from build123d import *

# Parameters (mm, degrees)
F1_DEPTH  = 150
F2_R      = 13.5859557656
F3_DEPTH  = 30
F3_FACE_R = 13.5859557656
F4_DEPTH  = 15
F4_TAPER  = -45


with BuildPart() as f1:
    # F0 (on Front) → F1 (new body)
    with BuildSketch(Plane.XZ):
        Polygon((-13.63390591, 4.962335928), (-13.63390591, -4.962335928), (-7.2544498107, -12.5650756531), (2.5194439792, -14.2884768348), (11.1144619307, -9.3261409068), (14.5088996214, 0), (11.1144619307, 9.3261409068), (2.5194439792, 14.2884768348), (-7.2544498107, 12.5650756531), align=None)
    extrude(amount=F1_DEPTH)

    # F2 (on face) → F3 (join)
    with BuildSketch(Plane.XZ.offset(150)):
        Circle(F2_R)
    extrude(amount=F3_DEPTH)

    # F3_face (on face) → F4 (join)
    with BuildSketch(Plane.XZ.offset(180)):
        Circle(F3_FACE_R)
    extrude(amount=F4_DEPTH, taper=F4_TAPER)


solid = f1.part
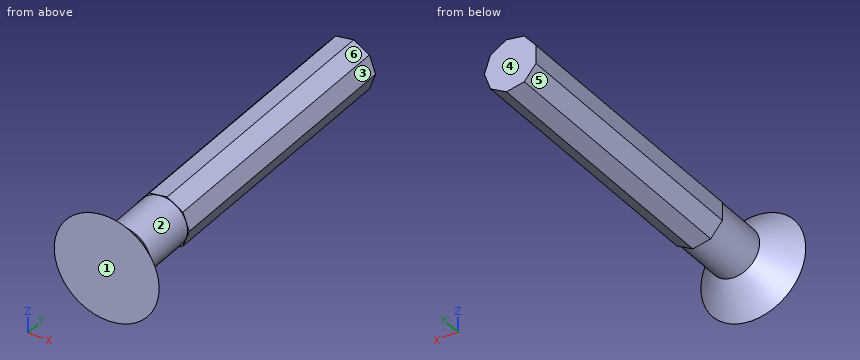
For this review, take the finished solid that the model builds, in its own axes (mm). Face numbers are marked on the shaded views. A direction names the side the tool comes from. Coordinates: 2 decimals unless noted, no trailing zeros. Write each loop counter-clockwise with the first axis right and the second up, starting at its lowest first coordinate (ties: lowest second). Pieces come first, ordered by that corner, then holes. Notation, with made-up numbers: (-37.75, 7) -> (-19.75, 7) arc R10 ccw to (-19.75, 15) -> close; hole circle Ø8 at (38.25, 14). An arc over 180 degrees is marked (long way). Write each question's results on one line, items separated by ' | '. Start each with the question number.
1) Consider section B-B (x = 0). Write out the cut boundary in (y, z), plus the area to 3 significant figures.
2) Wall thickness on L1, parallel to X at y = -178.5, z = -1; L2, parallel to Y at x = 14.5, z = 18.5; L3, parallel to Z at x = -5, y = -153.5: over which ranges is each line inside the solid? List them lowest first. Write a range as [from, to].
3) For the marked faces 5 and 6, list the 3-axis set-ups (+Z, -Z, +X, -X, +Y, -Y) from which the entire face can be reached by the end or side of a thin tool; tool diameter is ignored.
4) Insertion check: pin 1 (11 mm diameter, centred on y = -60, z = 0.5, fed in from -X); pin 2 (5 mm diameter, centred on x = -5, y = -147, fed in from -Z); pin 3 (10 mm diameter, centred on x = 20, y = -97.5, fed in from -Z); pin 4 (5 mm diameter, centred on x = 12, y = -112.5, fed in from +Z). Each pin has a flat end and moves straight along its axis. Give the tip position at first contact, or say it passes through.
5) Consider section A-A (y = -63.5). Write out the cut boundary in (x, z).
6) The part is to be moulded in two halves that separate along Y. For the marked faces 1, 2, 3 and 4, say which applies: +Y half, -Y half, draft (parallel to the pull), parting line (faces both ways), or undercut.
Geometry says:
1) outline: (-195, -28.59) -> (-180, -13.59) -> (-150, -13.59) -> (-150, -13.84) -> (0, -13.84) -> (0, 13.84) -> (-150, 13.84) -> (-150, 13.59) -> (-180, 13.59) -> (-195, 28.59) -> close | area: 5,600 mm^2
2) L1: [-13.55, 13.55] | L2: [-195, -189.92] | L3: [-12.63, 12.63]
3) face 5: -Z, -X, +Y | face 6: +Z, +X, +Y
4) pin 1: x = -13.63 | pin 2: z = -13.4 | pin 3: through | pin 4: z = 10.26
5) outline: (-13.63, -4.96) -> (-7.25, -12.57) -> (2.52, -14.29) -> (11.11, -9.33) -> (14.51, 0) -> (11.11, 9.33) -> (2.52, 14.29) -> (-7.25, 12.57) -> (-13.63, 4.96) -> close
6) face 1: -Y half | face 2: undercut | face 3: draft | face 4: +Y half
